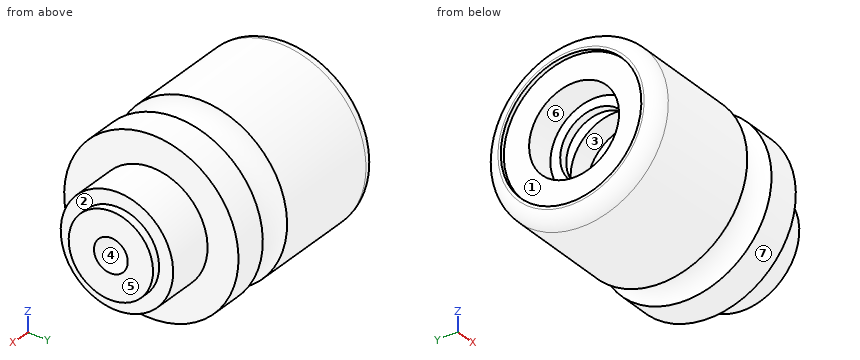
```python
from build123d import *

# Parameters (mm, degrees)
F4_R = 5


with BuildPart() as f2:
    # F0 (on Front) → F2 (revolve)
    with BuildSketch(Plane.XZ):
        with BuildLine():
            Line((0, 31), (0, 0))
            Line((0, 0), (88, 0))
            Line((88, 0), (88, 15))
            Line((88, 15), (85, 15))
            Line((85, 15), (85, 20))
            Line((85, 20), (68, 20))
            Line((68, 20), (68, 31))
            Line((68, 31), (56, 31))
            ThreePointArc((56, 31), (50, 25), (44, 31))
            Line((44, 31), (0, 31))
        make_face()
    revolve(axis=Axis((63.740881, 0, 0), (1, 0, 0)))

    # F1 (on Front) → F3 (revolve, cut)
    with BuildSketch(Plane.XZ):
        Polygon((1.5, 25), (0, 25), (0, 0), (88, 0), (88, 6), (30, 6), (30, 16), (22, 16), (22, 20.5), (15, 20.5), (15, 12.5), (12, 12.5), (12, 16), (1.5, 16), align=None)
    revolve(axis=Axis((-14.931626, 0, 0), (-1, 0, 0)), mode=Mode.SUBTRACT)

    # F4
    f4_edges = [f2.edges().sort_by_distance(p)[0] for p in [
        (0, 0, -31),
    ]]
    fillet(f4_edges, radius=F4_R)


solid = f2.part
```
Geometry: final body of the model. Coordinates: model frame, mm. Face numbers are marked on the shaded views. A direction names the side the tool comes from. Give positions to 0.01 mm unless a question says otherwise; leave off trailing zeros. Write each loop counter-clockwise with the first axis right and the second up, starting at its lowest first coordinate (ties: lowest second). Pieces come first, ordered by that corner, then holes.
1. Draft query along Z for the marked faces 5, 6 and 7. Return one class per face: released by +Z, released by -Z, zero draft, split by the parting line, or undercut.
2. Section query A-A, the plane x = 13. Return loops of the section in (y, z), then the cut area to 3 significant figures.
3. Reachability of the marked faces 1, 2, 3 and 4 from +Z, -Z, +X, -X, +Y, -Y: full face, straight path, thin tool, end or side. Return the list, or none.
4. Section query B-B, the plane x = 54. Return loops of the section in (y, z).
5. Line query: probe 1 along Y at (x, z) = (26.75, 0); probe 2 along Y at (x, z) = (74, 0); probe 3 along X at (y, z) = (6, 12). Output: solid intervals per line, ascending.
6. Pin query (flat end, axial travel): P1, Ø10, axis at x = 28, z = -12, coming from the -Y side; P2, Ø9.5, axis at y = 0, z = 0, coming from the -X side; P3, Ø2, axis at x = 75, y = -17, coming from the +Z side; P4, Ø1, axis at x = 31.5, z = 11, coming from the -Y side. Return the tip coordinate at first contact, or that it passes through.
Computed:
1. face 5: zero draft
1. face 6: undercut
1. face 7: split by the parting line
2. outline: circle Ø62 at (0, 0); hole circle Ø25 at (0, 0)
2. area: 2,530 mm2
3. face 1: -X
3. face 2: +X
3. face 3: none
3. face 4: +X, -X
4. outline: circle Ø53.06 at (0, 0); hole circle Ø12 at (0, 0)
5. probe 1: y = -31 to -16, 16 to 31
5. probe 2: y = -20 to -6, 6 to 20
5. probe 3: x = 12 to 15, 30 to 88
6. P1: stops at y = -30.2
6. P2: passes through
6. P3: stops at z = 12
6. P4: stops at y = -29.17
